Work out the finished part from the listing and answer in its coordinate system (mm). Coordinates: 2 decimals unless noted, no trailing zeros. Order: outer loops, then holes, each group sorted by start corner. A loop starts at its lowest first (then second) coordinate and runs counter-clockwise, first axis right, second up. Notation, with made-up numbers: M -5,-20 L 28,-20 A18 ccw 28,1 Z; hole C -31,24.25 d11. An arc over 180 degrees is marked long. Use a Markdown table: item, result.
from build123d import *

# Parameters (mm, degrees)
F0_W     = 19.05
F0_H     = 146.05
F1_DEPTH = 304.8
F4_DEPTH = 304.8
F6_DEPTH = 304.8
F7_W     = 12.7
F7_H     = 146.05
F8_DEPTH = 12.7


with BuildPart() as f1:
    # F0 (on Front) → F1 (new body)
    with BuildSketch(Plane.XZ):
        with Locations((9.525, 73.025)):
            Rectangle(F0_W, F0_H)
    extrude(amount=F1_DEPTH)

    # F3 (on Front) → F4 (cut)
    with BuildSketch(Plane.XZ):
        Polygon((19.05, 124.6124), (24.139026, 124.6124), (24.139026, 153.1874), (14.2875, 153.1874), (14.2875, 143.6624), (19.05, 142.604067), (19.05, 139.429067), (14.2875, 138.370733), (14.2875, 135.195733), (19.05, 134.1374), align=None)
    extrude(amount=F4_DEPTH, mode=Mode.SUBTRACT)

    # F5 (on Front) → F6 (cut)
    with BuildSketch(Plane.XZ):
        Polygon((24.139026, -7.1374), (24.139026, 21.4376), (19.05, 21.4376), (19.05, 11.9126), (14.2875, 10.854267), (14.2875, 7.679267), (19.05, 6.620933), (19.05, 3.445933), (14.2875, 2.3876), (14.2875, -7.1374), align=None)
    extrude(amount=F6_DEPTH, mode=Mode.SUBTRACT)

    # F7 (on offset) → F8 (cut)
    with BuildSketch(Plane.XZ.offset(25.4)):
        with Locations((21.1455, 73.025)):
            Rectangle(F7_W, F7_H)
    extrude(amount=-F8_DEPTH, mode=Mode.SUBTRACT)


solid = f1.part
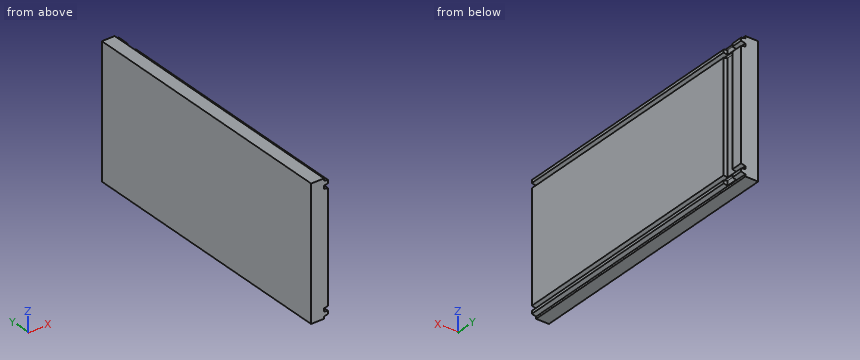
1. Section A-A on y = -250 is taken. Determine the outline of the cut face in (x, z), then the cut area to 3 significant figures.
Answers below:
| item | result |
|---|---|
| outline | M 0,0 L 14.29,0 L 14.29,2.39 L 19.05,3.45 L 19.05,6.62 L 14.29,7.68 L 14.29,10.85 L 19.05,11.91 L 19.05,134.14 L 14.29,135.2 L 14.29,138.37 L 19.05,139.43 L 19.05,142.6 L 14.29,143.66 L 14.29,146.05 L 0,146.05 Z |
| area | 2,710 mm² |
2. Flat-ended cylindrical pins translate along their axes: P1, Ø10, axis at x = 15.5, z = 110.5, coming from the +Y side; P2, Ø1.6, axis at y = -118.5, z = 9.5, coming from the +X side; P3, Ø4, axis at y = -20, z = 142, coming from the +X side. Find the tip coordinate at first contact, or state that the pin passes through.
Answers below:
| item | result |
|---|---|
| P1 | y = 0 |
| P2 | x = 14.29 |
| P3 | x = 14.8 |
3. Find the intervals of material crossed by probe 1 along Z at (x, y) = (15, -282); probe 2 along Y at (x, z) = (15, 31.5); probe 3 along Z at (x, y) = (17, -269.5), in increasing order.
Answers below:
| item | result |
|---|---|
| probe 1 | 2.55 to 7.52, 11.01 to 135.04, 138.53 to 143.5 |
| probe 2 | -304.8 to -25.4, -12.7 to 0 |
| probe 3 | 2.99 to 7.08, 11.46 to 134.59, 138.97 to 143.06 |
